from build123d import *

# Parameters (mm, degrees)
EXTRUDE6_DEPTH               = 3.162924
EXTRUDE6_2_DEPTH             = 3.162924
EXTRUDE6_3_DEPTH             = 3.162924
EXTRUDE6_4_DEPTH             = 3.162924
EXTRUDE6_5_DEPTH             = 3.162924
EXTRUDE6_6_DEPTH             = 3.162924
EXTRUDE7_START               = -2.752923646
EXTRUDE7_DEPTH               = 2.752923646
EXTRUDE1_DEPTH               = 2.165
EXTRUDE1_DEPTH_BACK          = 6.095
SKETCH3_R                    = 1.945
F_1_0_1_DIAMETER_HOLE1_D     = 1
F_1_0_1_DIAMETER_HOLE1_DEPTH = 13.97
F_1_0_1_DIAMETER_HOLE1_TIP   = 0.30043031


# Read off the part's stored shape, not the designer's step: Extrude7
with BuildPart() as part:
    # Sketch7 → Extrude6 (new body)
    with BuildSketch(Plane.XY):
        with BuildLine():
            Line((-5.535, -12.32), (-5.535, -7.224956165))
            Line((-5.535, -7.224956165), (-7.165, -6.314002227))
            Line((-7.165, -6.314002227), (-7.165, -7.17281133))
            ThreePointArc((-7.165, -7.17281133), (-6.454703172, -7.883108158), (-7.165, -8.593404986))
            Line((-7.165, -8.593404986), (-7.165, -12.32))
            Line((-7.165, -12.32), (-6.77, -12.32))
            Line((-6.77, -12.32), (-6.77, -17.360738904))
            Line((-6.77, -17.360738904), (-6.510329667, -18.42))
            Line((-6.510329667, -18.42), (-6.189670333, -18.42))
            Line((-6.189670333, -18.42), (-5.93, -17.360738904))
            Line((-5.93, -17.360738904), (-5.93, -12.32))
            Line((-5.93, -12.32), (-5.535, -12.32))
        make_face()
    extrude(amount=-EXTRUDE6_DEPTH)


with BuildPart() as body_2:
    # Sketch7 → Extrude6 2 (new body)
    with BuildSketch(Plane.XY):
        with BuildLine():
            Line((-4.625, -7.733525542), (-4.625, -12.32))
            Line((-4.625, -12.32), (-4.23, -12.32))
            Line((-4.23, -12.32), (-4.23, -17.360738904))
            Line((-4.23, -17.360738904), (-3.970329667, -18.42))
            Line((-3.970329667, -18.42), (-3.649670333, -18.42))
            Line((-3.649670333, -18.42), (-3.39, -17.360738904))
            Line((-3.39, -17.360738904), (-3.39, -12.32))
            Line((-3.39, -12.32), (-2.995, -12.32))
            Line((-2.995, -12.32), (-2.995, -8.535310619))
            ThreePointArc((-2.995, -8.535310619), (-3.582478148, -8.288826526), (-4.149861063, -7.999065227))
            Line((-4.149861063, -7.999065227), (-4.625, -7.733525542))
        make_face()
    extrude(amount=-EXTRUDE6_2_DEPTH)


with BuildPart() as body_3:
    # Sketch7 → Extrude6 3 (new body)
    with BuildSketch(Plane.XY):
        with BuildLine():
            Line((-0.455, -12.32), (-0.455, -9.067822531))
            ThreePointArc((-0.455, -9.067822531), (-1.276005531, -8.983751864), (-2.085, -8.82051612))
            Line((-2.085, -8.82051612), (-2.085, -12.32))
            Line((-2.085, -12.32), (-1.69, -12.32))
            Line((-1.69, -12.32), (-1.69, -17.360738904))
            Line((-1.69, -17.360738904), (-1.430329667, -18.42))
            Line((-1.430329667, -18.42), (-1.109670333, -18.42))
            Line((-1.109670333, -18.42), (-0.85, -17.360738904))
            Line((-0.85, -17.360738904), (-0.85, -12.32))
            Line((-0.85, -12.32), (-0.455, -12.32))
        make_face()
    extrude(amount=-EXTRUDE6_3_DEPTH)


with BuildPart() as body_4:
    # Sketch7 → Extrude6 4 (new body)
    with BuildSketch(Plane.XY):
        with BuildLine():
            Line((4.625, -12.32), (4.625, -7.733525542))
            Line((4.625, -7.733525542), (4.149861063, -7.999065227))
            ThreePointArc((4.149861063, -7.999065227), (3.582478148, -8.288826526), (2.995, -8.535310619))
            Line((2.995, -8.535310619), (2.995, -12.32))
            Line((2.995, -12.32), (3.39, -12.32))
            Line((3.39, -12.32), (3.39, -17.360738904))
            Line((3.39, -17.360738904), (3.649670333, -18.42))
            Line((3.649670333, -18.42), (3.970329667, -18.42))
            Line((3.970329667, -18.42), (4.23, -17.360738904))
            Line((4.23, -17.360738904), (4.23, -12.32))
            Line((4.23, -12.32), (4.625, -12.32))
        make_face()
    extrude(amount=-EXTRUDE6_4_DEPTH)


with BuildPart() as body_5:
    # Sketch7 → Extrude6 5 (new body)
    with BuildSketch(Plane.XY):
        with BuildLine():
            Line((0.455, -9.067822531), (0.455, -12.32))
            Line((0.455, -12.32), (0.85, -12.32))
            Line((0.85, -12.32), (0.85, -17.360738904))
            Line((0.85, -17.360738904), (1.109670333, -18.42))
            Line((1.109670333, -18.42), (1.430329667, -18.42))
            Line((1.430329667, -18.42), (1.69, -17.360738904))
            Line((1.69, -17.360738904), (1.69, -12.32))
            Line((1.69, -12.32), (2.085, -12.32))
            Line((2.085, -12.32), (2.085, -8.82051612))
            ThreePointArc((2.085, -8.82051612), (1.276005531, -8.983751864), (0.455, -9.067822531))
        make_face()
    extrude(amount=-EXTRUDE6_5_DEPTH)


with BuildPart() as body_6:
    # Sketch7 → Extrude6 6 (new body)
    with BuildSketch(Plane.XY):
        Polygon((5.535, -7.224956165), (5.535, -12.32), (5.93, -12.32), (5.93, -17.360738904), (6.189670333, -18.42), (6.510329667, -18.42), (6.77, -17.360738904), (6.77, -12.32), (7.165, -12.32), (7.165, -6.314002227), align=None)
    extrude(amount=-EXTRUDE6_6_DEPTH)


with BuildPart() as extrude7_tool:
    # Extrude7 outline → Extrude7 (new body)
    with BuildSketch(Plane.XY.offset(EXTRUDE7_START)):
        with BuildLine():
            Line((-5.93, -17.360738904), (-5.93, -12.32))
            Line((-5.93, -12.32), (-5.535, -12.32))
            Line((-5.535, -12.32), (-5.535, -7.224956165))
            Line((-5.535, -7.224956165), (-7.165, -6.314002227))
            Line((-7.165, -6.314002227), (-7.165, -7.17281133))
            ThreePointArc((-7.165, -7.17281133), (-6.454703172, -7.883108158), (-7.165, -8.593404986))
            Line((-7.165, -8.593404986), (-7.165, -12.32))
            Line((-7.165, -12.32), (-6.77, -12.32))
            Line((-6.77, -12.32), (-6.77, -17.360738904))
            Line((-6.77, -17.360738904), (-6.510329667, -18.42))
            Line((-6.510329667, -18.42), (-6.189670333, -18.42))
            Line((-6.189670333, -18.42), (-5.93, -17.360738904))
        make_face()
        Polygon((6.77, -17.360738904), (6.77, -12.32), (7.165, -12.32), (7.165, -6.314002227), (5.535, -7.224956165), (5.535, -12.32), (5.93, -12.32), (5.93, -17.360738904), (6.189670333, -18.42), (6.510329667, -18.42), align=None)
        with BuildLine():
            Line((4.23, -17.360738904), (4.23, -12.32))
            Line((4.23, -12.32), (4.625, -12.32))
            Line((4.625, -12.32), (4.625, -7.733525542))
            Line((4.625, -7.733525542), (4.149861063, -7.999065227))
            ThreePointArc((4.149861063, -7.999065227), (3.582478148, -8.288826526), (2.995, -8.535310619))
            Line((2.995, -8.535310619), (2.995, -12.32))
            Line((2.995, -12.32), (3.39, -12.32))
            Line((3.39, -12.32), (3.39, -17.360738904))
            Line((3.39, -17.360738904), (3.649670333, -18.42))
            Line((3.649670333, -18.42), (3.970329667, -18.42))
            Line((3.970329667, -18.42), (4.23, -17.360738904))
        make_face()
        with BuildLine():
            Line((1.69, -17.360738904), (1.69, -12.32))
            Line((1.69, -12.32), (2.085, -12.32))
            Line((2.085, -12.32), (2.085, -8.82051612))
            ThreePointArc((2.085, -8.82051612), (1.276005531, -8.983751864), (0.455, -9.067822531))
            Line((0.455, -9.067822531), (0.455, -12.32))
            Line((0.455, -12.32), (0.85, -12.32))
            Line((0.85, -12.32), (0.85, -17.360738904))
            Line((0.85, -17.360738904), (1.109670333, -18.42))
            Line((1.109670333, -18.42), (1.430329667, -18.42))
            Line((1.430329667, -18.42), (1.69, -17.360738904))
        make_face()
        with BuildLine():
            Line((-0.85, -17.360738904), (-0.85, -12.32))
            Line((-0.85, -12.32), (-0.455, -12.32))
            Line((-0.455, -12.32), (-0.455, -9.067822531))
            ThreePointArc((-0.455, -9.067822531), (-1.276005531, -8.983751864), (-2.085, -8.82051612))
            Line((-2.085, -8.82051612), (-2.085, -12.32))
            Line((-2.085, -12.32), (-1.69, -12.32))
            Line((-1.69, -12.32), (-1.69, -17.360738904))
            Line((-1.69, -17.360738904), (-1.430329667, -18.42))
            Line((-1.430329667, -18.42), (-1.109670333, -18.42))
            Line((-1.109670333, -18.42), (-0.85, -17.360738904))
        make_face()
        with BuildLine():
            Line((-3.39, -17.360738904), (-3.39, -12.32))
            Line((-3.39, -12.32), (-2.995, -12.32))
            Line((-2.995, -12.32), (-2.995, -8.535310619))
            ThreePointArc((-2.995, -8.535310619), (-3.582478148, -8.288826526), (-4.149861063, -7.999065227))
            Line((-4.149861063, -7.999065227), (-4.625, -7.733525542))
            Line((-4.625, -7.733525542), (-4.625, -12.32))
            Line((-4.625, -12.32), (-4.23, -12.32))
            Line((-4.23, -12.32), (-4.23, -17.360738904))
            Line((-4.23, -17.360738904), (-3.970329667, -18.42))
            Line((-3.970329667, -18.42), (-3.649670333, -18.42))
            Line((-3.649670333, -18.42), (-3.39, -17.360738904))
        make_face()
    extrude(amount=EXTRUDE7_DEPTH)


with BuildPart() as part_1:
    add(part.part)

    # Extrude7: cut by extrude7_tool
    add(extrude7_tool.part, mode=Mode.SUBTRACT)



with BuildPart() as body_2_1:
    add(body_2.part)

    # Extrude7: cut by extrude7_tool
    add(extrude7_tool.part, mode=Mode.SUBTRACT)


with BuildPart() as body_3_1:
    add(body_3.part)

    # Extrude7: cut by extrude7_tool
    add(extrude7_tool.part, mode=Mode.SUBTRACT)


with BuildPart() as body_4_1:
    add(body_4.part)

    # Extrude7: cut by extrude7_tool
    add(extrude7_tool.part, mode=Mode.SUBTRACT)


with BuildPart() as body_5_1:
    add(body_5.part)

    # Extrude7: cut by extrude7_tool
    add(extrude7_tool.part, mode=Mode.SUBTRACT)


with BuildPart() as body_6_1:
    add(body_6.part)

    # Extrude7: cut by extrude7_tool
    add(extrude7_tool.part, mode=Mode.SUBTRACT)


with BuildPart() as part_2:
    add(part_1.part)

    add(body_2_1.part)  # Extrude1 merges body 2

    add(body_3_1.part)  # Extrude1 merges body 3

    add(body_4_1.part)  # Extrude1 merges body 4

    add(body_5_1.part)  # Extrude1 merges body 5

    add(body_6_1.part)  # Extrude1 merges body 6
    # Sketch3 → Extrude1 (add, two sides: drawn at the far end of the back side and taken through both)
    with BuildSketch(Plane.XY.offset(-EXTRUDE1_DEPTH_BACK)):
        with BuildLine():
            Line((4.149861063, -7.999065227), (13.199056425, -2.941764516))
            ThreePointArc((13.199056425, -2.941764516), (14.925, 0), (13.199056425, 2.941764516))
            Line((13.199056425, 2.941764516), (4.149861063, 7.999065227))
            ThreePointArc((4.149861063, 7.999065227), (0, 9.08), (-4.149861063, 7.999065227))
            Line((-4.149861063, 7.999065227), (-13.199056425, 2.941764516))
            ThreePointArc((-13.199056425, 2.941764516), (-14.925, 0), (-13.199056425, -2.941764516))
            Line((-13.199056425, -2.941764516), (-4.149861063, -7.999065227))
            ThreePointArc((-4.149861063, -7.999065227), (0, -9.08), (4.149861063, -7.999065227))
        make_face()
        with Locations((11.555, 0)):
            Circle(SKETCH3_R, mode=Mode.SUBTRACT)
        with Locations((-11.555, 0)):
            Circle(SKETCH3_R, mode=Mode.SUBTRACT)
    extrude(amount=EXTRUDE1_DEPTH + EXTRUDE1_DEPTH_BACK)

    # Sketch5 → Cut-Revolve1 (revolve, cut)
    with BuildSketch(Plane(origin=(0, 0, 0), x_dir=(0, 0, -1), z_dir=(1, 0, 0)), mode=Mode.PRIVATE) as cut_revolve1_sk:
        Polygon((4.310187736, -16.063245386), (4.310187736, -7.724967149), (6.095, -6.063245386), (6.095, -16.063245386), align=None)
    revolve(cut_revolve1_sk.sketch.rotate(Axis((0, 0, 0), (0, 0, 1)), 270), axis=Axis((0, 0, 0), (0, 0, 1)), mode=Mode.SUBTRACT)

    # Sketch8 → Revolve1 (revolve)
    with BuildSketch(Plane(origin=(0, 0, 0), x_dir=(0, 0, -1), z_dir=(1, 0, 0)), mode=Mode.PRIVATE) as revolve1_sk:
        Polygon((0, 0), (0, 20.522309629), (-1.878035446, 20.522309629), (-1.878035446, 17.921716672), (-2.411490412, 12.387121404), (-1.649027846, 12.387121404), (-1.649027846, 9.857883061), (-2.165, 9.342309629), (-2.165, 0), align=None)
    revolve(revolve1_sk.sketch.rotate(Axis((0, 20.522309629, 0), (0, 1, 0)), 180), axis=Axis((0, 20.522309629, 0), (0, 1, 0)))

    # Ø1.0 (1) Diameter Hole1
    with Locations(Plane.ZX.offset(20.522309629)):
        with Locations((0, 0)):
            Hole(F_1_0_1_DIAMETER_HOLE1_D / 2, depth=F_1_0_1_DIAMETER_HOLE1_DEPTH)
            with Locations((0, 0, -(F_1_0_1_DIAMETER_HOLE1_DEPTH + F_1_0_1_DIAMETER_HOLE1_TIP / 2))):  # 118° drill point
                Cone(0, F_1_0_1_DIAMETER_HOLE1_D / 2, F_1_0_1_DIAMETER_HOLE1_TIP, mode=Mode.SUBTRACT)


solid = part_2.part
For this review, take the finished solid that the model builds, in its own axes (mm). A direction names the side the tool comes from. Give positions to 0.01 mm unless a question says otherwise; leave off trailing zeros. Loops run counter-clockwise (first coordinate to the right, second up) from the corner with the lowest first, then second, coordinate; pieces in that order, holes last.
Item 1: Insertion check: pin 1 (12 mm diameter, centred on x = 5.5, y = -7, fed in from +Z) (3 decimals); pin 2 (0.5 mm diameter, centred on x = -4, y = -15.5, fed in from -Z); pin 3 (0.5 mm diameter, centred on y = -15, z = -3, fed in from +X). Each pin has a flat end and moves straight along its axis. Give the tip position at first contact, or say it passes through.
Item 2: Tool access review of faces 4 (the flat face through (6, -11, -3.163)), 5 (the flat face through (0, 0, 2.165)), 6 (the flat face through (8, 0, -4.31)), 7 (the cylindrical face through (-0.488, 13.44, 0.108)): name each direction out of +Z, -Z, +X, -X, +Y, -Y from which nothing blocks a thin tool from reaching the whole face with its end or side.
Item 3: For line 1 along X through (y, z) = (0, -2) (3 decimals); line 2 along Y through (x, z) = (-0.5, -0.75); line 3 along Y through (x, z) = (12, -3.5), list the stretches that pass through material, from the lowest coordinate up.
Item 4: Take a section at B-B, the plane y = -15. State the section outline as (x, z) points, and give its area (3 significant figures).
Item 5: Take a section at D-D, the plane z = 1.25. Give the number of separate pieces and of enclosed holes in the cut face, and give its area (3 significant figures).
Item 6: Draft analysis for pull direction Z (two halves, no side actions). For faces 1 (the flat face through (-8.738, -5.435, -1.118)), 2 (the flat face through (6, -11, -2.753)), 3 (the conical face through (-0.08, 6.3, -0.02)), state which applies: +Z half, -Z half, draft (parallel to the pull), parting line (faces both ways), or undercut.
Item 7: Take a section at A-A, the plane y = 0. State the section outline as (x, z) points (3 decimals).
Item 8: Take a section at C-C, the plane x = 12.5. State the section outline as (y, z) points (3 decimals).
Calculated:
1. pin 1: stops at z = 2.165
1. pin 2: stops at z = -3.16
1. pin 3: stops at x = 6.77
2. face 4: -Z, +X, -Y
2. face 5: +Z, +X, -X, -Y
2. face 6: -Z
2. face 7: +Y
3. line 1: x = -14.925 to -13.5, -9.61 to 9.61, 13.5 to 14.925
3. line 2: y = -9.07 to 20.52
3. line 3: y = -3.61 to -1.89, 1.89 to 3.61
4. outline: (-6.77, -3.16) - (-5.93, -3.16) - (-5.93, -2.75) - (-6.77, -2.75) - close; (-4.23, -3.16) - (-3.39, -3.16) - (-3.39, -2.75) - (-4.23, -2.75) - close; (-1.69, -3.16) - (-0.85, -3.16) - (-0.85, -2.75) - (-1.69, -2.75) - close; (0.85, -3.16) - (1.69, -3.16) - (1.69, -2.75) - (0.85, -2.75) - close; (3.39, -3.16) - (4.23, -3.16) - (4.23, -2.75) - (3.39, -2.75) - close; (5.93, -3.16) - (6.77, -3.16) - (6.77, -2.75) - (5.93, -2.75) - close
4. area: 2.07 mm2
5. separate pieces: 1
5. enclosed holes: 2
5. area: 368 mm2
6. face 1: draft
6. face 2: +Z half
6. face 3: undercut
7. outline: (-14.925, -4.31) - (-13.5, -4.31) - (-13.5, 2.165) - (-14.925, 2.165) - close; (-9.61, -4.31) - (-7.725, -4.31) - (-6.063, -6.095) - (6.063, -6.095) - (7.725, -4.31) - (9.61, -4.31) - (9.61, 2.165) - (-9.61, 2.165) - close; (13.5, -4.31) - (14.925, -4.31) - (14.925, 2.165) - (13.5, 2.165) - close
8. outline: (-3.332, -4.31) - (-1.7, -4.31) - (-1.7, 2.165) - (-3.332, 2.165) - close; (1.7, -4.31) - (3.332, -4.31) - (3.332, 2.165) - (1.7, 2.165) - close
